Could you check a few things on this model? Use its own coordinates, in mm. Give positions to 0.01 mm unless a question says otherwise; leave off trailing zeros. Loops run counter-clockwise (first coordinate to the right, second up) from the corner with the lowest first, then second, coordinate; pieces in that order, holes last. Notation, with made-up numbers: M -18,53.25 L 13,53.25 A27 cw 13,89.25 Z; hole C 32,0 d8. An arc over 180 degrees is marked long. Use CSV: the item, a comma, the result in double quotes.
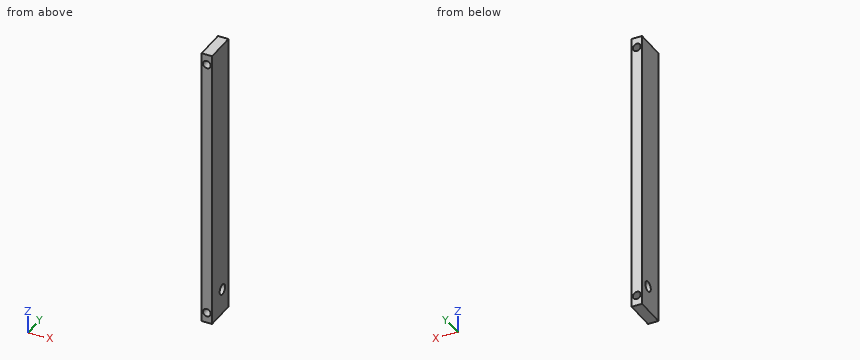
```python
from build123d import *

# Parameters (mm, degrees)
SKETCH1_W           = 6.35
SKETCH1_H           = 19.05
BOSS_EXTRUDE1_DEPTH = 172.72
SKETCH4_R           = 3.175000102
CUT_EXTRUDE3_DEPTH  = 25.4
SKETCH2_R           = 2.3368
CUT_EXTRUDE4_DEPTH  = 174.883361481


with BuildPart() as part:
    # Sketch1 → Boss-Extrude1 (new body)
    with BuildSketch(Plane.XY):
        with Locations((-3.175, 9.525)):
            Rectangle(SKETCH1_W, SKETCH1_H)
    extrude(amount=BOSS_EXTRUDE1_DEPTH)

    # Sketch4 → Cut-Extrude3 (cut)
    with BuildSketch(Plane(origin=(0, 0, 0), x_dir=(0, 0, -1), z_dir=(1, 0, 0))):
        with Locations((-15.24, 12.065)):
            Circle(SKETCH4_R)
    extrude(amount=-CUT_EXTRUDE3_DEPTH, mode=Mode.SUBTRACT)

    # Sketch2 → Cut-Extrude4 (cut, through all)
    with BuildSketch(Plane(origin=(0, 19.05, 0), x_dir=(1, 0, 0), z_dir=(0, 1, 0))):
        with Locations(Location((-3.175, -166.37, 0), (0, 0, 270))):
            Circle(SKETCH2_R)
        with Locations(Location((-3.175, -6.35, 0), (0, 0, 270))):
            Circle(SKETCH2_R)
    extrude(amount=-CUT_EXTRUDE4_DEPTH, mode=Mode.SUBTRACT)


solid = part.part
```
1. I want a section at A-A, the plane z = 15.24. List the corners of the cut face in (x, y) for me, then the cut area to 3 significant figures.
Outcome:
outline,"M -6.35,0 L 0,0 L 0,8.89 L -6.35,8.89 Z; M -6.35,15.24 L 0,15.24 L 0,19.05 L -6.35,19.05 Z"
area,"80.6 mm2"
2. I want a section at C-C, the plane y = 3. List the corners of the cut face in (x, z) for me (3 decimals), then the cut area to 3 significant figures.
Outcome:
outline,"M -6.35,0 L 0,0 L 0,172.72 L -6.35,172.72 Z; hole C -3.175,6.35 d4.674; hole C -3.175,166.37 d4.674"
area,"1,060 mm2"
3. I'm going to push a flat-ended pin straight in: pin 1 Ø3 at (x, z) = (-3, 141) entering from -Y. Where does the tip first touch, or does it pass through?
Outcome:
pin 1,"y = 0"
4. Please list where these lines run through material, in increasing order: line 1 (Z direction, x = -3, y = 5.5); line 2 (Z direction, x = -3.5, y = 2); line 3 (X direction, y = 9.75, z = 166.37).
Outcome:
line 1,"0 to 4.02, 8.68 to 164.04, 168.7 to 172.72"
line 2,"0 to 4.04, 8.66 to 164.06, 168.68 to 172.72"
line 3,"-6.35 to -5.51, -0.84 to 0"
5. I want a section at B-B, the plane z = 166.37. List the corners of the cut face in (x, y) for me, then the cut area to 3 significant figures.
Outcome:
outline,"M -6.35,0 L -5.51,0 L -5.51,19.05 L -6.35,19.05 Z; M -0.84,0 L 0,0 L 0,19.05 L -0.84,19.05 Z"
area,"31.9 mm2"
